```python
from build123d import *

# Parameters (mm, degrees)
F0_R     = 5
F1_DEPTH = 2
F2_R     = 4
F3_DEPTH = 6.1
F4_R     = 2.5
F5_DEPTH = 4.5
F7_D     = 2
F7_DEPTH = 4
F7_TIP   = 0.600860619


with BuildPart() as f1:
    # F0 (on Top) → F1 (new body)
    with BuildSketch(Plane.XY):
        Circle(F0_R)
    extrude(amount=F1_DEPTH)

    # F2 (on face) → F3 (join)
    with BuildSketch(Plane.XY.offset(2)):
        Circle(F2_R)
    extrude(amount=F3_DEPTH)

    # F4 (on face) → F5 (join)
    with BuildSketch(Plane.XY.offset(8.1)):
        Circle(F4_R)
    extrude(amount=F5_DEPTH)

    # F7
    with Locations(Plane.XY.offset(12.6)):
        with Locations((0, 0)):
            Hole(F7_D / 2, depth=F7_DEPTH)
            with Locations((0, 0, -(F7_DEPTH + F7_TIP / 2))):  # 118° drill point
                Cone(0, F7_D / 2, F7_TIP, mode=Mode.SUBTRACT)


solid = f1.part
```
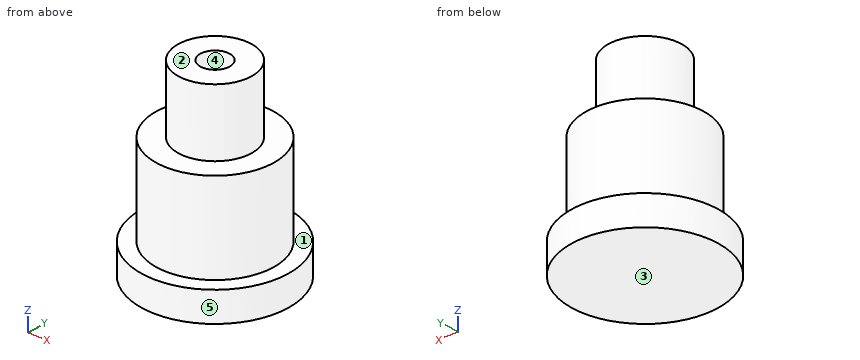
Work out the finished part from the listing and answer in its coordinate system (mm). Face numbers are marked on the shaded views. A direction names the side the tool comes from. Coordinates: 2 decimals unless noted, no trailing zeros. Write each loop counter-clockwise with the first axis right and the second up, starting at its lowest first coordinate (ties: lowest second). Pieces come first, ordered by that corner, then holes.
Q1. A cutting plane is placed at B-B, the plane y = -2.75. Give the vertices of the cut face in (x, z), then the cut area to 3 significant figures.
Q2. A cutting plane is placed at D-D, the plane x = 2.25. Give the vertices of the cut face in (y, z), then the cut area to 3 significant figures.
Q3. A cutting plane is placed at A-A, the plane x = -3. Give the vertices of the cut face in (y, z).
Q4. A cutting plane is placed at C-C, the plane y = 2. Give the vertices of the cut face in (x, z).
Q5. Each of these flat-tipped pins is pushed along its axis until it touches: pin 1 Ø1.5 at (x, z) = (-2.5, 2.5) entering from -Y; pin 2 Ø3 at (x, z) = (-1, 9.5) entering from -Y; pin 3 Ø3 at (y, z) = (-1.5, 10) entering from -X; pin 4 Ø5 at (x, y) = (-3, 0) entering from +Z. Where does it stop, or does it pass through?
Q6. Find the intervals of material crossed by line 1 (Y direction, x = 0, z = 11.1); line 2 (Z direction, x = 1.5, y = -3.5); line 3 (Z direction, x = -3.5, y = 3.25), in increasing order.
Q7. Determine the mould class of the marked faces 3, 4 and 5 for opening direction X: released by +X, released by -X, zero draft, split by the parting line, or undercut.
Q8. Which of the six approach directions +Z, -Z, +X, -X, +Y, -Y give full straight-line access (tool end or side, diameter ignored) to the marked faces 1 and 2?
Findings below:
1. outline: (-4.18, 0) - (4.18, 0) - (4.18, 2) - (2.9, 2) - (2.9, 8.1) - (-2.9, 8.1) - (-2.9, 2) - (-4.18, 2) - close
1. area: 52.1 mm2
2. outline: (-4.47, 0) - (4.47, 0) - (4.47, 2) - (3.31, 2) - (3.31, 8.1) - (1.09, 8.1) - (1.09, 12.6) - (-1.09, 12.6) - (-1.09, 8.1) - (-3.31, 8.1) - (-3.31, 2) - (-4.47, 2) - close
2. area: 68.0 mm2
3. outline: (-4, 0) - (4, 0) - (4, 2) - (2.65, 2) - (2.65, 8.1) - (-2.65, 8.1) - (-2.65, 2) - (-4, 2) - close
4. outline: (-4.58, 0) - (4.58, 0) - (4.58, 2) - (3.46, 2) - (3.46, 8.1) - (1.5, 8.1) - (1.5, 12.6) - (-1.5, 12.6) - (-1.5, 8.1) - (-3.46, 8.1) - (-3.46, 2) - (-4.58, 2) - close
5. pin 1: stops at y = -4.61
5. pin 2: stops at y = -3.97
5. pin 3: stops at x = -2.5
5. pin 4: stops at z = 12.6
6. line 1: y = -2.5 to -1, 1 to 2.5
6. line 2: z = 0 to 8.1
6. line 3: z = 0 to 2
7. face 3: zero draft
7. face 4: undercut
7. face 5: split by the parting line
8. face 1: +Z
8. face 2: +Z, +X, -X, +Y, -Y
